Here's the drawing with two shaded views (mm, measured from the low corner). I have some questions. A direction names the side the tool comes from. Give positions to 0.01 mm unless a question says otherwise; leave off trailing zeros. Write each loop counter-clockwise with the first axis right and the second up, starting at its lowest first coordinate (ties: lowest second). Pieces come first, ordered by that corner, then holes. Notation, with made-up numbers: M -5.75,86.25 L 4.25,86.25 A27 cw 4.25,114.25 Z; hole C 4.5,27.5 d3. An arc over 180 degrees is marked long. Use one line per item in the form item = value. Start each with the question number.
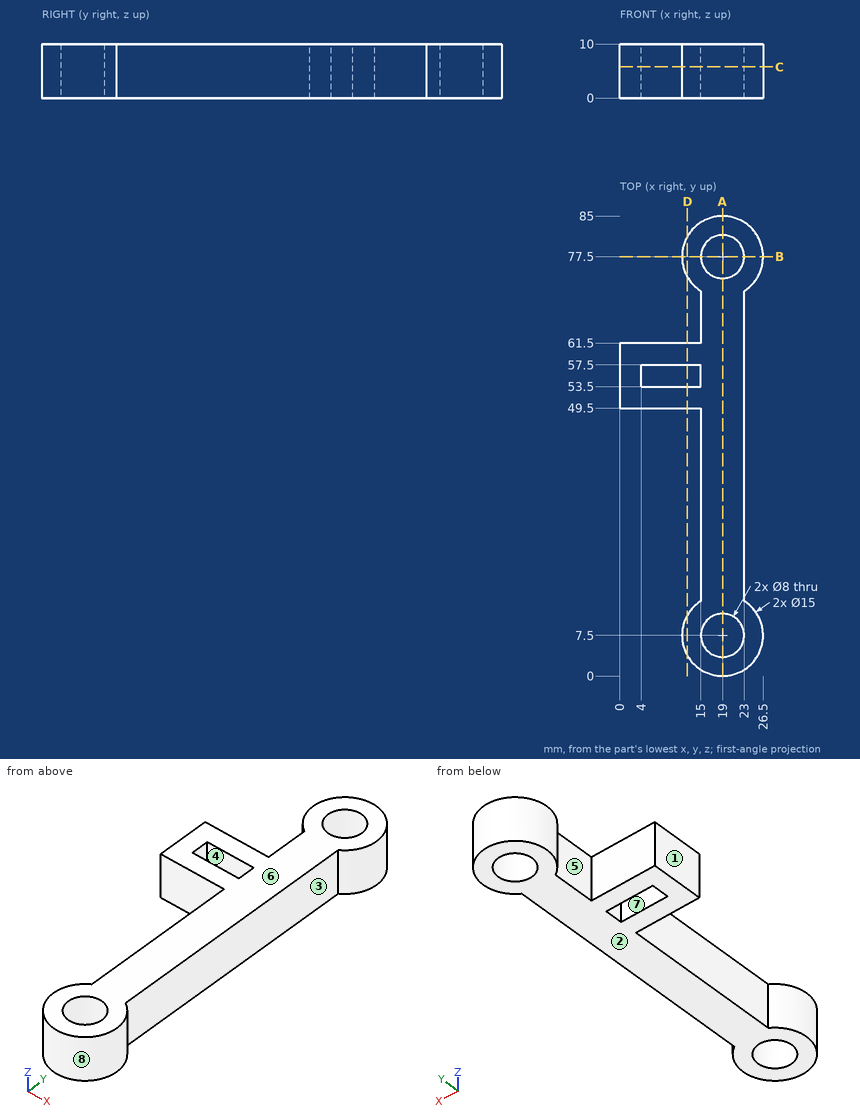
1) Suppose I cut it at B-B, the plane y = 77.5. List the corners of the cut face in (x, z) for me.
2) On a 3-axis mill with a long thin cutter (end or side, diameter ignored), from which of +Z, -Z, +X, -X, +Y, -Y can I reach the whole of each face in a straight line? I mean the marked faces 1, 2, 3, 4 and 5. Say none if no direction works.
3) Will these pins go through, and if not, where does the flat tip stop? P1, Ø4, axis at x = 16, z = 2, coming from the -Y side; P2, Ø5, axis at y = 67, z = 4, coming from the -X side; P3, Ø3, axis at x = 11.5, z = 6.5, coming from the -Y side; P4, Ø7, axis at x = 19, y = 7.5, coming from the +Z side.
4) Suppose I cut it at C-C, the plane z = 5.75. List the corners of the cut face in (x, y) for me, and give its area (3 significant figures).
5) Please list where these lines run through material, in increasing order: line 1 (Y direction, x = 8, z = 4); line 2 (Y direction, x = 13, z = 9); line 3 (Y direction, x = 21.5, z = 5.75).
6) Suppose I cut it at A-A, the plane x = 19. List the corners of the cut face in (y, z) for me, and give its area (3 significant figures).
7) Thinking about a two-plate mould opening in X: for the marked faces 6, 7 and 8, which applies, released by +X, released by -X, zero draft, split by the parting line, or undercut?
8) Suppose I cut it at D-D, the plane x = 12.5. List the corners of the cut face in (y, z) for me.
Checks:
q1.outline = M 11.5,0 L 15,0 L 15,10 L 11.5,10 Z; M 23,0 L 26.5,0 L 26.5,10 L 23,10 Z
q2.face_1 = +Z, -Z, -X, +Y, -Y
q2.face_2 = -Z, +X, -X, +Y, -Y
q2.face_3 = +Z, -Z, +X
q2.face_4 = +Z, -Z
q2.face_5 = +Z, -Z, -X
q3.P1 = 0.07
q3.P2 = 15
q3.P3 = 3
q3.P4 = through
q4.outline = M 0,49.5 L 15,49.5 L 15,13.84 A7.5 ccw long 23,13.84 L 23,71.16 A7.5 ccw long 15,71.16 L 15,61.5 L 0,61.5 Z; hole M 4,53.5 L 15,53.5 L 15,57.5 L 4,57.5 Z; hole C 19,7.5 d8; hole C 19,77.5 d8
q4.area = 835 mm^2
q5.line_1 = 49.5 to 53.5, 57.5 to 61.5
q5.line_2 = 3 to 12, 49.5 to 53.5, 57.5 to 61.5, 73 to 82
q5.line_3 = 0.43 to 4.38, 10.62 to 74.38, 80.62 to 84.57
q6.outline = M 0,0 L 3.5,0 L 3.5,10 L 0,10 Z; M 11.5,0 L 73.5,0 L 73.5,10 L 11.5,10 Z; M 81.5,0 L 85,0 L 85,10 L 81.5,10 Z
q6.area = 690 mm^2
q7.face_6 = zero draft
q7.face_7 = undercut
q7.face_8 = split by the parting line
q8.outline = M 3.76,0 L 11.24,0 L 11.24,10 L 3.76,10 Z; M 49.5,0 L 53.5,0 L 53.5,10 L 49.5,10 Z; M 57.5,0 L 61.5,0 L 61.5,10 L 57.5,10 Z; M 73.76,0 L 81.24,0 L 81.24,10 L 73.76,10 Z
